from build123d import *

# Parameters (mm, degrees)
BOSS_EXTRUDE2_DEPTH = 12.7
SKETCH3_R           = 12
CUT_EXTRUDE1_DEPTH  = 15.24
SKETCH5_R           = 3.96875
CUT_EXTRUDE3_DEPTH  = 26.4
SKETCH4_R           = 5
CUT_EXTRUDE2_DEPTH  = 26.4
CUT_EXTRUDE4_DEPTH  = 11.1125
CUT_EXTRUDE5_DEPTH  = 11.1125
SKETCH10_R          = 12.7
CUT_EXTRUDE6_DEPTH  = 5.3975
CUT_EXTRUDE7_REACH  = 29.328
SKETCH12_W          = 38.1
SKETCH12_H          = 15.875
CUT_EXTRUDE8_REACH  = 31.596
SKETCH15_W          = 38.1
SKETCH15_H          = 15.875
FILLET1_R           = 3.175
FILLET2_R           = 3.175
FILLET3_R           = 6.35
CHAMFER1_SIZE       = 0.635


with BuildPart() as part:
    # Sketch2 → Boss-Extrude2 (new body, symmetric)
    with BuildSketch(Plane(origin=(0, 0, 0), x_dir=(1, 0, 0), z_dir=(0, 1, 0))):
        with BuildLine():
            Line((-58.565346794, 6.551716506), (-2.085197783, 73.494164894))
            ThreePointArc((-2.085197783, 73.494164894), (9.165477674, 76.485932244), (15.840147634, 66.947737915))
            Line((15.840147634, 66.947737915), (15.874997849, 0.008264886))
            ThreePointArc((15.874997849, 0.008264886), (10.578143579, -11.83716619), (-1.7859375, -15.77422113))
            Line((-1.7859375, -15.77422113), (-51.943, -10.095501523))
            ThreePointArc((-51.943, -10.095501523), (-60.240451667, -3.755459003), (-58.565346794, 6.551716506))
        make_face()
    extrude(amount=BOSS_EXTRUDE2_DEPTH, both=True)

    # Sketch3 → Cut-Extrude1 (cut)
    with BuildSketch(Plane.XZ.offset(12.7)):
        Circle(SKETCH3_R)
    extrude(amount=-CUT_EXTRUDE1_DEPTH, mode=Mode.SUBTRACT)

    # Sketch5 → Cut-Extrude3 (cut, through all)
    with BuildSketch(Plane(origin=(0, 12.7, 0), x_dir=(1, 0, 0), z_dir=(0, 1, 0))):
        with Locations((-50.8, 0)):
            Circle(SKETCH5_R)
        with Locations((5.680149011, 66.942448388)):
            Circle(SKETCH5_R)
    extrude(amount=-CUT_EXTRUDE3_DEPTH, mode=Mode.SUBTRACT)

    # Sketch4 → Cut-Extrude2 (cut, through all)
    with BuildSketch(Plane(origin=(0, 12.7, 0), x_dir=(1, 0, 0), z_dir=(0, 1, 0))):
        Circle(SKETCH4_R)
    extrude(amount=-CUT_EXTRUDE2_DEPTH, mode=Mode.SUBTRACT)

    # Sketch6 → Cut-Extrude4 (cut)
    with BuildSketch(Plane(origin=(0, 12.7, 0), x_dir=(1, 0, 0), z_dir=(0, 1, 0))):
        with BuildLine():
            Line((-39.764503985, 23.911604457), (-16.032698846, 52.039454127))
            ThreePointArc((-16.032698846, 52.039454127), (-11.636571539, 54.278149682), (-6.964480572, 52.69408558))
            ThreePointArc((-6.964480572, 52.69408558), (-0.854842234, 49.048416159), (6.166313709, 47.898652971))
            ThreePointArc((6.166313709, 47.898652971), (10.759647518, 46.098936994), (12.678367748, 41.55402712))
            Line((12.678367748, 41.55402712), (12.688909771, 21.305156508))
            ThreePointArc((12.688909771, 21.305156508), (10.136411612, 16.212500271), (4.527793308, 15.215607538))
            ThreePointArc((4.527793308, 15.215607538), (-10.578143579, 11.83716619), (-15.626938173, -2.7954299))
            ThreePointArc((-15.626938173, -2.7954299), (-17.245628646, -8.257136186), (-22.592088443, -10.223290312))
            Line((-22.592088443, -10.223290312), (-26.354947036, -9.797264189))
            ThreePointArc((-26.354947036, -9.797264189), (-30.656406746, -7.381661273), (-31.930429027, -2.615681803))
            ThreePointArc((-31.930429027, -2.615681803), (-33.099153125, 7.041485631), (-38.883371679, 14.862586231))
            ThreePointArc((-38.883371679, 14.862586231), (-41.231270715, 19.201372144), (-39.764503985, 23.911604457))
        make_face()
    extrude(amount=-CUT_EXTRUDE4_DEPTH, mode=Mode.SUBTRACT)

    # Sketch8 → Cut-Extrude5 (cut)
    with BuildSketch(Plane.XZ.offset(12.7)):
        with BuildLine():
            Line((-26.354947036, 9.797264189), (-22.592088443, 10.223290312))
            ThreePointArc((-22.592088443, 10.223290312), (-17.245628646, 8.257136186), (-15.626938173, 2.7954299))
            ThreePointArc((-15.626938173, 2.7954299), (-10.578143579, -11.83716619), (4.527793308, -15.215607538))
            ThreePointArc((4.527793308, -15.215607538), (10.136411612, -16.212500271), (12.688909771, -21.305156508))
            Line((12.688909771, -21.305156508), (12.678367748, -41.55402712))
            ThreePointArc((12.678367748, -41.55402712), (10.759647518, -46.098936994), (6.166313709, -47.898652971))
            ThreePointArc((6.166313709, -47.898652971), (-0.854842234, -49.048416159), (-6.964480572, -52.69408558))
            ThreePointArc((-6.964480572, -52.69408558), (-11.636571539, -54.278149682), (-16.032698846, -52.039454127))
            Line((-16.032698846, -52.039454127), (-39.764503985, -23.911604457))
            ThreePointArc((-39.764503985, -23.911604457), (-41.231270715, -19.201372144), (-38.883371679, -14.862586231))
            ThreePointArc((-38.883371679, -14.862586231), (-33.099153125, -7.041485631), (-31.930429027, 2.615681803))
            ThreePointArc((-31.930429027, 2.615681803), (-30.656406746, 7.381661273), (-26.354947036, 9.797264189))
        make_face()
    extrude(amount=-CUT_EXTRUDE5_DEPTH, mode=Mode.SUBTRACT)

    # Sketch10 → Cut-Extrude6 (cut)
    with BuildSketch(Plane(origin=(0, 12.7, 0), x_dir=(1, 0, 0), z_dir=(0, 1, 0))):
        Circle(SKETCH10_R)
    extrude(amount=-CUT_EXTRUDE6_DEPTH, mode=Mode.SUBTRACT)

    # Sketch12 → Cut-Extrude7 (cut, up to next)
    with BuildSketch(Plane(origin=(17.337923239, 0, -47.474487057), x_dir=(0.939319277, 0, 0.34304416), z_dir=(-0.34304416, 0, 0.939319277)), mode=Mode.PRIVATE) as cut_extrude7_sk1:
        with Locations((-17.6287425, 0)):
            Rectangle(SKETCH12_W, SKETCH12_H)
    cut_extrude7_tool1 = extrude(cut_extrude7_sk1.sketch, amount=-CUT_EXTRUDE7_REACH, mode=Mode.PRIVATE) & part.part
    add(cut_extrude7_tool1.solids().sort_by_distance((0.778906, 0, -53.521924))[0], mode=Mode.SUBTRACT)

    # Sketch15 → Cut-Extrude8 (cut, up to next)
    with BuildSketch(Plane(origin=(-30.583679643, 0, 12.166341096), x_dir=(0.369631792, 0, 0.929178314), z_dir=(-0.929178314, 0, 0.369631792)), mode=Mode.PRIVATE) as cut_extrude8_sk1:
        with Locations((-18.777295017, 0)):
            Rectangle(SKETCH15_W, SKETCH15_H)
    cut_extrude8_tool1 = extrude(cut_extrude8_sk1.sketch, amount=CUT_EXTRUDE8_REACH, mode=Mode.PRIVATE) & part.part
    add(cut_extrude8_tool1.solids().sort_by_distance((-37.524365, 0, -5.281114))[0], mode=Mode.SUBTRACT)

    # Fillet1
    fillet1_edges = [part.edges().sort_by_distance(p)[0] for p in [
        (-30.656406746, 1.5875, 7.381661273),
        (-33.099153125, 1.5875, -7.041485631),
        (-41.231270715, 1.5875, -19.201372144),
        (-27.898601415, 1.5875, -37.975529292),
        (-11.636571539, 1.5875, -54.278149682),
        (-0.854842234, 1.5875, -49.048416159),
        (10.759647518, 1.5875, -46.098936994),
        (12.68363876, 1.5875, -31.429591814),
        (10.136411612, 1.5875, -16.212500271),
        (-10.578143579, 1.5875, -11.83716619),
        (-17.245628646, 1.5875, 8.257136186),
        (-24.473517739, 1.5875, 10.01027725),
    ]]
    fillet(fillet1_edges, radius=FILLET1_R)

    # Fillet2
    fillet2_edges = [part.edges().sort_by_distance(p)[0] for p in [
        (-17.245628646, -1.5875, 8.257136186),
        (-10.578143579, -1.5875, -11.83716619),
        (10.136411612, -1.5875, -16.212500271),
        (12.68363876, -1.5875, -31.429591814),
        (10.759647518, -1.5875, -46.098936994),
        (-0.854842234, -1.5875, -49.048416159),
        (-11.636571539, -1.5875, -54.278149682),
        (-27.898601415, -1.5875, -37.975529292),
        (-41.231270715, -1.5875, -19.201372144),
        (-33.099153125, -1.5875, -7.041485631),
        (-30.656406746, -1.5875, 7.381661273),
        (-24.473517739, -1.5875, 10.01027725),
    ]]
    fillet(fillet2_edges, radius=FILLET2_R)

    # Fillet3
    fillet3_edges = [part.edges().sort_by_distance(p)[0] for p in [
        (0.778905577, 7.9375, -53.521924216),
        (0.778905577, -7.9375, -53.521924216),
        (-37.524364844, 7.9375, -5.281114224),
        (-37.524364844, -7.9375, -5.281114224),
    ]]
    fillet(fillet3_edges, radius=FILLET3_R)

    # Chamfer1
    chamfer1_edges = [part.edges().sort_by_distance(p)[0] for p in [
        (-12, -12.7, 0),
    ]]
    chamfer(chamfer1_edges, length=CHAMFER1_SIZE)


solid = part.part
Geometry check sheet. Reference: the model listing, model coordinates, mm. A direction names the side the tool comes from. Give positions to 0.01 mm unless a question says otherwise; leave off trailing zeros. Write each loop counter-clockwise with the first axis right and the second up, starting at its lowest first coordinate (ties: lowest second). Pieces come first, ordered by that corner, then holes. Notation, with made-up numbers: (41.25, 30) - (66.25, 30) arc R17 cw to (66.25, 52) - close; hole circle Ø4 at (87.25, 82.5). An arc over 180 degrees is marked (long way). Put each result on its own line as item: value.
1. Set-up check for faces 1 (the cylindrical face through (-17.303, -8.787, 8.317)), 2 (the flat face through (-47, -7.938, 2)), 3 (the flat face through (-28.065, 8.787, -37.779)): record each of +Z, -Z, +X, -X, +Y, -Y from which the full face is reachable in a straight line by a thin tool's end or side.
Ans:
face 1: -Y
face 2: +Z, -X
face 3: +Y
2. Sectioned sample at A-A, the plane x = -50.8. Enter the section's corners in (y, z).
Ans:
outline: (-12.7, -15.76) - (-7.94, -15.76) - (-7.94, -3.97) - (-12.7, -3.97) - close; (-12.7, 3.97) - (-7.94, 3.97) - (-7.94, 10.22) - (-12.7, 10.22) - close; (7.94, -15.76) - (12.7, -15.76) - (12.7, -3.97) - (7.94, -3.97) - close; (7.94, 3.97) - (12.7, 3.97) - (12.7, 10.22) - (7.94, 10.22) - close
3. Draft check along X on faces 4 (the flat face through (7, 7.938, -63)), 5 (the cylindrical face through (-41.238, -8.787, -19.272)), 6 (the flat face through (0.57, 0.02, -53.6)). Enter one of: +X half, -X half, draft (parallel to the pull), parting line (faces both ways), or undercut.
Ans:
face 4: draft
face 5: undercut
face 6: +X half
4. Thickness scan on line 1 (X direction, y = 10.2, z = 0) (3 decimals); line 2 (Y direction, x = -46.5, z = 8.5); line 3 (Z direction, x = -6, y = 10.75). Record the ranges inside material, lowest first.
Ans:
line 1: x = -60.96 to -54.769, -46.831 to -31.75, -15.875 to -12.7, 12.7 to 15.875
line 2: y = -12.7 to -7.94, 7.94 to 12.7
line 3: z = -68.85 to -51.89, -14.7 to -11.19, 11.19 to 15.3
5. Go/stop test with flat-tipped pins: pin 1 (2 mm diameter, centred on x = -11.5, y = 3.5, fed in from +Z); pin 2 (4 mm diameter, centred on y = 2.5, z = -5.5, fed in from -X); pin 3 (13 mm diameter, centred on x = 0, z = 0, fed in from +Y); pin 4 (7 mm diameter, centred on x = 5.68, z = -66.94, fed in from -Y). Record where each tip stops, or that it passes through.
Ans:
pin 1: stops at z = 14.79
pin 2: stops at x = -38.65
pin 3: stops at y = 7.3
pin 4: passes through
6. Sectioned sample at B-B, the plane y = -6.75. Give the number of separate pieces and of enclosed holes in the cut face, plus the area to 3 significant figures.
Ans:
separate pieces: 1
enclosed holes: 2
area: 1,140 mm²
